CAD build for the part. Positions are in the model's coordinates, mm. Coordinates: 2 decimals unless noted, no trailing zeros. Order: outer loops, then holes, each group sorted by start corner. A loop starts at its lowest first (then second) coordinate and runs counter-clockwise, first axis right, second up. Notation, with made-up numbers: M 27,5 L 71,5 A5 cw 71,12 Z; hole C 30.25,-9 d9. An arc over 180 degrees is marked long. Write item = value, one per line.
from build123d import *

# Parameters (mm, degrees)
SKETCH1_W           = 39
SKETCH1_H           = 39
SKETCH1_R           = 1.75
BOSS_EXTRUDE1_DEPTH = 4
SKETCH2_R           = 1.75
CUT_EXTRUDE1_DEPTH  = 11
FILLET1_R           = 1


with BuildPart() as part:
    # Sketch1 → Boss-Extrude1 (new body)
    with BuildSketch(Plane(origin=(0, 0, 0), x_dir=(1, 0, 0), z_dir=(0, 1, 0))):
        Rectangle(SKETCH1_W, SKETCH1_H)
        with Locations(Location((17, 17, 0), (0, 0, 270))):
            Circle(SKETCH1_R, mode=Mode.SUBTRACT)
        with Locations(Location((17, -17, 0), (0, 0, 270))):
            Circle(SKETCH1_R, mode=Mode.SUBTRACT)
        with Locations(Location((-17, -17, 0), (0, 0, 270))):
            Circle(SKETCH1_R, mode=Mode.SUBTRACT)
        with Locations(Location((-17, 17, 0), (0, 0, 270))):
            Circle(SKETCH1_R, mode=Mode.SUBTRACT)
    extrude(amount=BOSS_EXTRUDE1_DEPTH)

    # Sketch2 → Cut-Extrude1 (cut)
    with BuildSketch(Plane(origin=(0, 4, 0), x_dir=(1, 0, 0), z_dir=(0, 1, 0))):
        with Locations(Location((10, 10, 0), (0, 0, 270))):
            Circle(SKETCH2_R)
        with Locations(Location((10, -10, 0), (0, 0, 270))):
            Circle(SKETCH2_R)
        with Locations(Location((-10, -10, 0), (0, 0, 270))):
            Circle(SKETCH2_R)
        with Locations(Location((-10, 10, 0), (0, 0, 270))):
            Circle(SKETCH2_R)
    extrude(amount=-CUT_EXTRUDE1_DEPTH, mode=Mode.SUBTRACT)

    # Fillet1
    fillet1_edges = [part.edges().sort_by_distance(p)[0] for p in [
        (19.5, 2, 19.5),
        (-19.5, 2, 19.5),
        (-19.5, 2, -19.5),
        (19.5, 2, -19.5),
    ]]
    fillet(fillet1_edges, radius=FILLET1_R)


solid = part.part
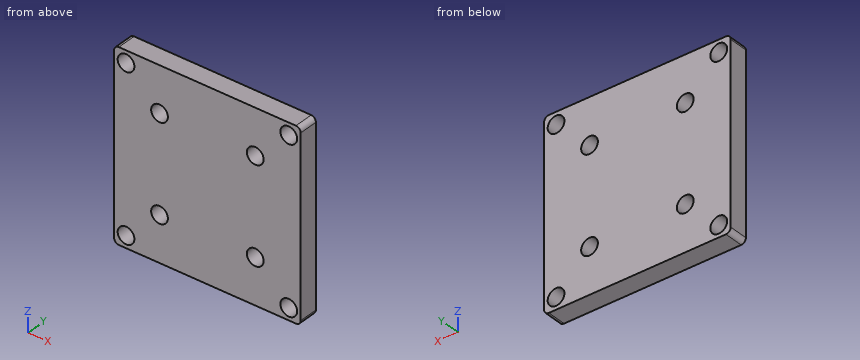
(1) Slice it at B-B, the plane z = 17. Write the cut outline in (x, y), then the cut area to 3 significant figures.
Evaluation:
outline = M -19.5,0 L -18.75,0 L -18.75,4 L -19.5,4 Z; M -15.25,0 L 15.25,0 L 15.25,4 L -15.25,4 Z; M 18.75,0 L 19.5,0 L 19.5,4 L 18.75,4 Z
area = 128 mm²
(2) Pin check, flat tip, straight feed: pin 1 Ø3 at (x, z) = (-10, 10) entering from -Y. Stop position of the tip, or through.
Evaluation:
pin_1 = through
(3) Wall check: line 1 (X direction, y = 1.35, z = -10); line 2 (X direction, y = 1.95, z = 17); line 3 (Z direction, x = 11, y = 3.5). Give the ranges that are in metal, low to high. Write a range as from..to.
Evaluation:
line_1 = -19.5..-11.75, -8.25..8.25, 11.75..19.5
line_2 = -19.5..-18.75, -15.25..15.25, 18.75..19.5
line_3 = -19.5..-11.44, -8.56..8.56, 11.44..19.5
(4) Slice it at A-A, the plane x = 17. Write the cut outline in (y, z), then the cut area to 3 significant figures.
Evaluation:
outline = M 0,-19.5 L 4,-19.5 L 4,-18.75 L 0,-18.75 Z; M 0,-15.25 L 4,-15.25 L 4,15.25 L 0,15.25 Z; M 0,18.75 L 4,18.75 L 4,19.5 L 0,19.5 Z
area = 128 mm²
(5) Slice it at C-C, the plane y = 0.7. State how many separate pieces and enclosed holes the cut face has, then the cut area to 3 significant figures.
Evaluation:
separate_pieces = 1
enclosed_holes = 8
area = 1,440 mm²
